Input: part model. Units: mm. Frame: model coordinates. Face numbers are marked on the shaded views. Coordinates: 2 decimals unless noted, no trailing zeros. Order: outer loops, then holes, each group sorted by start corner. A loop starts at its lowest first (then second) coordinate and runs counter-clockwise, first axis right, second up. Notation, with made-up numbers: (89, 8.25) -> (132, 8.25) arc R35 ccw to (132, 47.25) -> close; hole circle Ø10 at (54.25, 22.5). An arc over 180 degrees is marked (long way). Write each question's results on one line, items separated by ' | '.
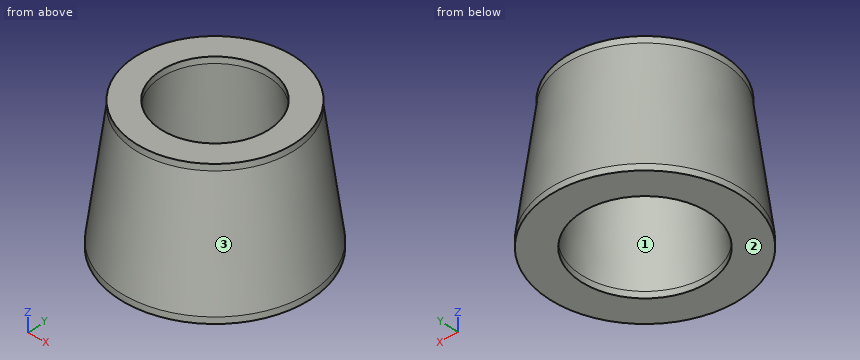
Autodesk Inventor part; units mm, degrees
ref_plane "Work Plane1" through (0, 0, 26.67) normal (0, 0, 1) x (1, 0, 0)
ref_plane "Work Plane2" through (0, 19.05, 26.67) normal (1, 0, 0) x (0, -1, 0)
ref_plane "YZ Plane" through (0, 0, 0) normal (1, 0, 0) x (0, 1, 0)
sketch "Sketch2" plane through (0, 0, 0) normal (0, 0, 1) x (1, 0, 0)
  circle A0 centre (0, 0) radius 19.05
  circle A1 centre (0, 0) radius 12.7
  dimension "d0" = 38.1
  dimension "d1" = 25.4
ref_plane "Work Plane1" through (0, 0, 26.67) normal (0, 0, 1) x (1, 0, 0)
sketch "Sketch3" plane through (0, 0, 26.67) normal (0, 0, 1) x (1, 0, 0)
  circle A0 centre (0, 0) radius 15.875
  circle A1 centre (0, 0) radius 10.795
  dimension "d5" = 31.75
  dimension "d6" = 21.59
extrude "Extrusion2" add sketch "Sketch3" against normal blind 1.27
extrude "Extrusion3" add sketch "Sketch2" along normal blind 1.27
sketch "Sketch4" plane through (0, 0, 26.67) normal (0, 0, 1) x (1, 0, 0)
  circle A0 centre (0, 0) radius 19.05
  line L0 (0, 19.05) -> (0, 0) construction
ref_plane "Work Plane2" through (0, 19.05, 26.67) normal (1, 0, 0) x (0, -1, 0)
sketch "Sketch5" plane through (0, 19.05, 26.67) normal (1, 0, 0) x (0, -1, 0)
  line L0 (34.925, 1.27) -> (3.175, 1.27)
  line L1 (0, 25.4) -> (38.1, 25.4)
  line L2 (3.175, 1.27) -> (0, 25.4)
  line L3 (8.255, 1.27) -> (29.845, 1.27)
  line L4 (31.75, 25.4) -> (6.35, 25.4)
  line L5 (6.35, 1.27) -> (6.35, 25.4)
  line L6 (6.35, 25.4) -> (0, 25.4)
  line L7 (8.255, 1.27) -> (3.175, 1.27)
  line L8 (19.05, -0.091501) -> (19.05, 9.410296) construction
  point P0 (19.05, 26.67)
sketch "Sketch5 outline for Revolution1" plane through (0, 19.05, 26.67) normal (1, 0, 0) x (0, -1, 0)
  line L0 (0, 25.4) -> (3.175, 1.27)
  line L1 (6.35, 25.4) -> (0, 25.4)
  line L2 (8.255, 1.27) -> (6.35, 25.4)
  line L3 (3.175, 1.27) -> (8.255, 1.27)
revolve "Revolution1" add sketch "Sketch5 outline for Revolution1" angle 360 about axis through (0, 0, 26.761501) along (0, 0, -1)
properties part number "ecomake end part"
(1) Pin query (flat end, axial travel): P1, Ø4, axis at x = -1.5, z = 8.5, coming from the -Y side; P2, Ø1, axis at x = -6, z = 20.5, coming from the +Y side; P3, Ø1.5, axis at y = -11, z = 19.5, coming from the -X side; P4, Ø20.5, axis at x = 0, y = 0, coming from the -Z side. Return the tip coordinate at first contact, or that it passes through.
Return value:
P1: y = -18.33 | P2: y = 15.59 | P3: x = -13.14 | P4: through
(2) Cut plane C-C, the plane z = 11.5. Return loops of the section in (x, y), plus the area to 3 significant figures.
Return value:
outline: circle Ø35.41 at (0, 0); hole circle Ø23.78 at (0, 0) | area: 540 mm2
(3) Line query: line 1 along Y through (x, z) = (0, 0.4); line 2 along Y through (x, z) = (0, 25.85) (3 decimals). Output: solid intervals per line, ascending. Write a range as from..to.
Return value:
line 1: -19.05..-12.7, 12.7..19.05 | line 2: -15.875..-10.795, 10.795..15.875
(4) Cut plane D-D, the plane z = 14.5. Return loops of the section in (x, y).
Return value:
outline: circle Ø34.62 at (0, 0); hole circle Ø23.31 at (0, 0)
(5) Mould query, pull axis Y, two halves, no side actions, for the marked faces 1, 2 and 3. Classes: +Y half, -Y half, draft (parallel to the pull), parting line (faces both ways), or undercut.
Return value:
face 1: undercut | face 2: draft | face 3: parting line
(6) Cut plane A-A, the plane x = 0. Return loops of the section in (y, z) (3 decimals), plus the area to 3 significant figures.
Return value:
outline: (-19.05, 0) -> (-12.7, 0) -> (-12.7, 1.27) -> (-10.795, 25.4) -> (-10.795, 26.67) -> (-15.875, 26.67) -> (-15.875, 25.4) -> (-19.05, 1.27) -> close; (10.795, 25.4) -> (12.7, 1.27) -> (12.7, 0) -> (19.05, 0) -> (19.05, 1.27) -> (15.875, 25.4) -> (15.875, 26.67) -> (10.795, 26.67) -> close | area: 305 mm2
